Autodesk Inventor part; units mm, degrees
ref_plane "Work Plane3" through (0, 0, 0) normal (0, 1, 0) x (0, 0, 1)
ref_plane "YZ Plane" through (0, 0, 0) normal (1, 0, 0) x (0, 1, 0)
ref_plane "XY Plane" through (0, 0, 0) normal (0, 0, 1) x (1, 0, 0)
sketch "Sketch1" plane through (0, 0, 0) normal (0, 0, 1) x (1, 0, 0)
  circle A0 centre (0, 0) radius 12
  circle A1 centre (0, 0) radius 4
  line L0 (3.873, 1) -> (4.8, 1)
  line L1 (4.8, 1) -> (4.8, -1)
  line L2 (4.8, -1) -> (3.873, -1)
  circle A2 centre (0, 8) radius 2
  circle A3 centre (-6.9282, -4) radius 2
  circle A4 centre (6.9282, -4) radius 2
  point P0 (4.8, 0)
  point P1 (-4, 0)
  dimension "d0" = 24
  dimension "d1" = 8
  dimension "d2" = 2
  dimension "d3" = 8.8
  dimension "d4" = 4
  dimension "d5" = 8
  dimension "d8" = 360
extrude "Extrusion1" add sketch "Sketch1" along normal blind 10 contours A0 | A2 | A3 | A4
ref_plane "Work Plane3" through (0, 0, 0) normal (0, 1, 0) x (0, 0, 1)
ref_plane "Work Plane2" through (0, 0, 0) normal (0.866, -0.5, 0) x (0, 0, 1)
sketch "Sketch2" plane through (0, 0, 0) normal (0, 1, 0) x (0, 0, 1)
  line L0 (10, -12) -> (10, 12)
  line L1 (0, -12) -> (0, 12)
  line L2 (0, 12) -> (10, 12)
  line L3 (0, -12) -> (10, -12)
  point P0 (0, 0)
  point P1 (5, 0)
  point P2 (5, -12)
  point P3 (10, 0)
hole "Hole1" at (0, 0, 5) direction (0, -1, 0) diameter 2.459 end through all
sketch "Sketch3" plane through (0, 0, 0) normal (0.866, -0.5, 0) x (0, 0, 1)
  line L0 (0, -12) -> (0, 12)
  line L1 (0, -3.266) -> (0, -1.534)
  line L2 (0, -2.8025) -> (0, -3.266)
  line L3 (0, -1.0705) -> (0, -2.8025)
  line L4 (0, -1.534) -> (0, -1.0705)
  line L5 (0, 12) -> (10, 12)
  line L6 (0, -12) -> (10, -12)
  point P0 (0, 0)
  point P1 (0, 2)
  point P2 (0, -2)
  point P3 (0, 8.9282)
  point P4 (0, 4.9282)
  point P5 (0, -4.9282)
  point P6 (0, -8.9282)
  point P7 (5, 0)
  point P8 (5, -12)
  point P9 (0, 0)
hole "Hole2" at (0, 0, 5) direction (-0.866, 0.5, 0) diameter 2.459 end through all
hole "Hole3" at (0, 8, 0) at (-6.9282, -4, 0) at (6.9282, -4, 0) direction (0, 0, 1) diameter 3.242 end through all
ref_plane "Work Plane1" through (0, 0, 0) normal (-0.5, -0.866, 0) x (0, 0, 1)
properties part number "spiebaan mount 10 mm" material "Aluminum 6061"
Here's how the part is built. I have some questions about the finished solid (model axes, mm). A direction names the side the tool comes from. Round coordinates to 2 decimals unless told otherwise and drop trailing zeros. Write each loop counter-clockwise with the first axis right and the second up, starting at its lowest first coordinate (ties: lowest second). Pieces come first, ordered by that corner, then holes. Notation, with made-up numbers: (35.5, -4) -> (47.5, -4) arc R29 cw to (47.5, 22) -> close; hole circle Ø2 at (-29.5, 73.25). An arc over 180 degrees is marked (long way). One line per item, written item: value.
1) Suppose I cut it at A-A on x = 0. List the corners of the cut face in (y, z) for me, plus the area to 3 significant figures.
Filled sheet:
outline: (-12, 0) -> (-4, 0) -> (-4, 3.77) -> (-12, 3.77) -> close; (-12, 6.23) -> (-4, 6.23) -> (-4, 10) -> (-12, 10) -> close; (4, 0) -> (6.38, 0) -> (6.38, 10) -> (4, 10) -> close; (9.62, 0) -> (12, 0) -> (12, 10) -> (9.62, 10) -> close
area: 108 mm2
2) For faces 5 (the face through (-0.05, -7.96, 3.77)), 6 (the face through (4.3, 1, 4.9)), 7 (the face through (-3, 3, 10)), which set-ups out of +Z, -Z, +X, -X, +Y, -Y let a thin tool reach every point of the face, with its end or its side?
Filled sheet:
face 5: -Y
face 6: +Z, -Z
face 7: +Z, +X, -X, +Y, -Y
3) If I drill on line 1 (Y direction, x = 0, z = 7.25); line 2 (Y direction, x = -0.5, z = 8); line 3 (Z direction, x = 0, y = -5.75), over which ranges is the centre line in solid material (lowest first)? Write a range as [from, to].
Filled sheet:
line 1: y = [-12, -4], [4, 6.38], [9.62, 12]
line 2: y = [-11.99, -3.97], [3.97, 6.46], [9.54, 11.99]
line 3: z = [0, 3.77], [6.23, 10]
4) Suppose I cut it at B-B on y = 0. List the corners of the cut face in (x, z) for me, plus the area to 3 significant figures.
Filled sheet:
outline: (-12, 0) -> (-4, 0) -> (-4, 10) -> (-12, 10) -> close; (4.8, 0) -> (12, 0) -> (12, 10) -> (4.8, 10) -> close
area: 152 mm2
5) Suppose I cut it at D-D on x = 6. List the corners of the cut face in (y, z) for me.
Filled sheet:
outline: (-10.39, 0) -> (-5.33, 0) -> (-5.33, 10) -> (-10.39, 10) -> close; (-2.67, 0) -> (10.39, 0) -> (10.39, 10) -> (-2.67, 10) -> close
6) We'd pull the mould along X, two halves only. Please class faces 1 (the face through (-11.99, -0.53, 4.93)), 2 (the face through (4.8, 0, 5)), 3 (the face through (-3, 3, 0)), 4 (the face through (8.5, -4.4, 5.1)): released by +X, released by -X, zero draft, split by the parting line, or undercut.
Filled sheet:
face 1: split by the parting line
face 2: undercut
face 3: zero draft
face 4: undercut
7) I'm going to push flat-ended pins straight in: pin 1 Ø2.5 at (x, y) = (0, 8) entering from +Z; pin 2 Ø0.7 at (x, z) = (4, 2.5) entering from +Y; pin 3 Ø3 at (x, z) = (-5, 8.5) entering from -Y; pin 4 Ø3 at (y, z) = (-4, 4.5) entering from +X. Where does each tip first touch, or does it pass through?
Filled sheet:
pin 1: passes through
pin 2: stops at y = 11.43
pin 3: stops at y = -11.48
pin 4: stops at x = 11.74
8) Suppose I cut it at C-C on z = 5.5. List the corners of the cut face in (x, y) for me, plus the area to 3 significant figures.
Filled sheet:
outline: (-10.91, 5) arc R12 ccw to (-1.12, -11.95) -> (-1.12, -3.84) arc R4 cw to (-3.89, 0.95) -> close; (-9.79, 6.95) -> (-2.76, 2.89) arc R4 cw to (3.87, 1) -> (4.8, 1) -> (4.8, -1) -> (3.87, -1) arc R4 cw to (1.12, -3.84) -> (1.12, -11.95) arc R12 ccw (long way) to start; hole circle Ø3.24 at (-6.93, -4); hole circle Ø3.24 at (0, 8); hole circle Ø3.24 at (6.93, -4)
area: 340 mm2
